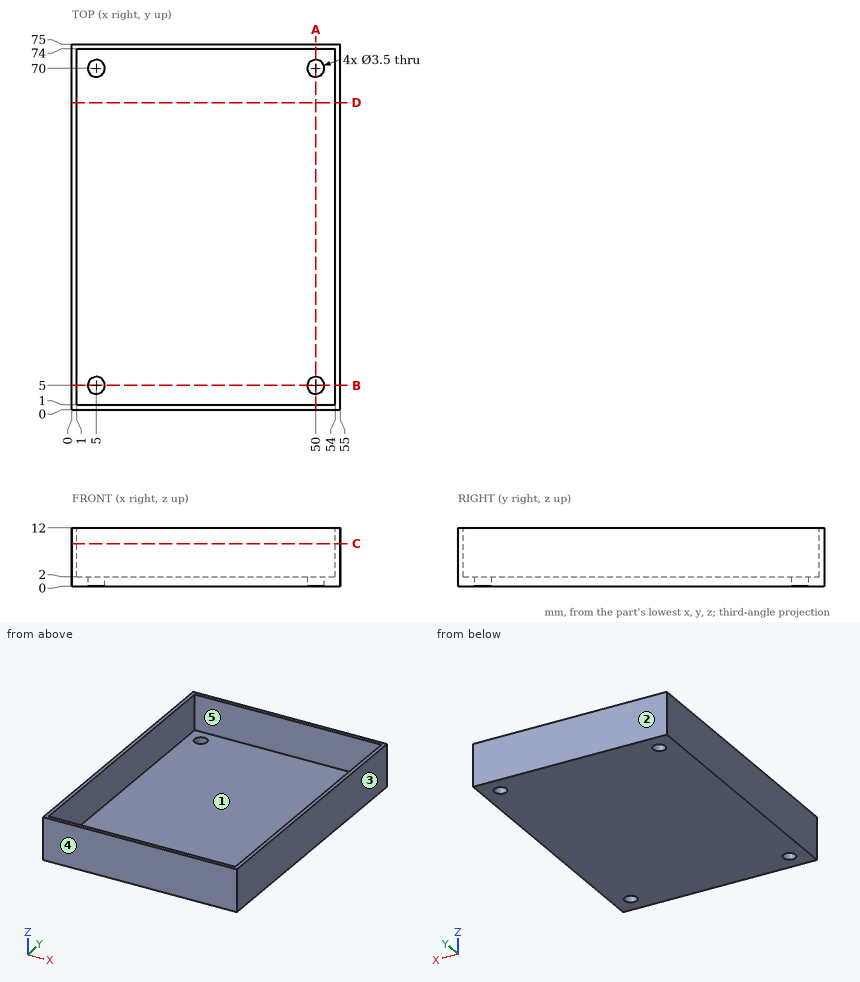
Job drawing, mm, ordinate dimensions from the low corner. One solid piece. A direction names the side the tool comes from. Round coordinates to 2 decimals unless told otherwise and drop trailing zeros. Loops run counter-clockwise (first coordinate to the right, second up) from the corner with the lowest first, then second, coordinate; pieces in that order, holes last. Notation, with made-up numbers: M 69.25,21 L 91.25,21 A22 ccw 91.25,53 Z; hole C 3,-24.5 d6. An arc over 180 degrees is marked long. Answer as CSV lines item,"result".
1. Flat gauge pins, fed straight in: P1, Ø3, axis at x = 48.5, y = 28, coming from the +Z side; P2, Ø1.5, axis at x = 11, z = 5.5, coming from the -Y side. Where does each tip first touch, or does it go through?
Resolved:
P1,"stops at z = 2"
P2,"stops at y = 0"
2. Cut at A-A on x = 50. Write the cut outline in (y, z).
Resolved:
outline,"M 0,0 L 3.25,0 L 3.25,2 L 1,2 L 1,12 L 0,12 Z; M 6.75,0 L 68.25,0 L 68.25,2 L 6.75,2 Z; M 71.75,0 L 75,0 L 75,12 L 74,12 L 74,2 L 71.75,2 Z"
3. Cut at C-C on z = 8.75. Write the cut outline in (x, y).
Resolved:
outline,"M 0,0 L 55,0 L 55,75 L 0,75 Z; hole M 1,1 L 54,1 L 54,74 L 1,74 Z"
4. 3-axis set-ups, long thin cutter, end or side, ignore diameter. For the marked faces 4 and 5: which of +Z, -Z, +X, -X, +Y, -Y reach the whole face in a straight line?
Resolved:
face 4,"+Z, -Z, +X, -X, -Y"
face 5,"+Z"
5. Two-plate mould, pull along X, no slides. Class the marked faces 1, 2 and 3: released by +X, released by -X, zero draft, split by the parting line, or undercut.
Resolved:
face 1,"undercut"
face 2,"zero draft"
face 3,"released by +X"
6. Cut at B-B on y = 5. Write the cut outline in (x, z), then the cut area to 3 significant figures.
Resolved:
outline,"M 0,0 L 3.25,0 L 3.25,2 L 1,2 L 1,12 L 0,12 Z; M 6.75,0 L 48.25,0 L 48.25,2 L 6.75,2 Z; M 51.75,0 L 55,0 L 55,12 L 54,12 L 54,2 L 51.75,2 Z"
area,"116 mm²"
7. Wall check: probe 1 along X at (y, z) = (70, 1.3); probe 2 along Y at (x, z) = (50, 0.85); probe 3 along X at (y, z) = (21, 3.5). Give the ranges that are in metal, low to high. Write a range as [from, to].
Resolved:
probe 1,"x = [0, 3.25], [6.75, 48.25], [51.75, 55]"
probe 2,"y = [0, 3.25], [6.75, 68.25], [71.75, 75]"
probe 3,"x = [0, 1], [54, 55]"
8. Cut at D-D on y = 63. Write the cut outline in (x, z), then the cut area to 3 significant figures.
Resolved:
outline,"M 0,0 L 55,0 L 55,12 L 54,12 L 54,2 L 1,2 L 1,12 L 0,12 Z"
area,"130 mm²"
